Drawing for the job (mm, zero at the part's lowest x, y, z). A direction names the side the tool comes from. Round coordinates to 2 decimals unless told otherwise and drop trailing zeros. Write each loop counter-clockwise with the first axis right and the second up, starting at its lowest first coordinate (ties: lowest second). Pieces come first, ordered by that corner, then holes. Notation, with made-up numbers: (6, 33) - (30, 33) arc R27 cw to (30, 54) - close; hole circle Ø7 at (-28, -40). An arc over 180 degrees is marked (long way). Answer in a Markdown table with one row per item.
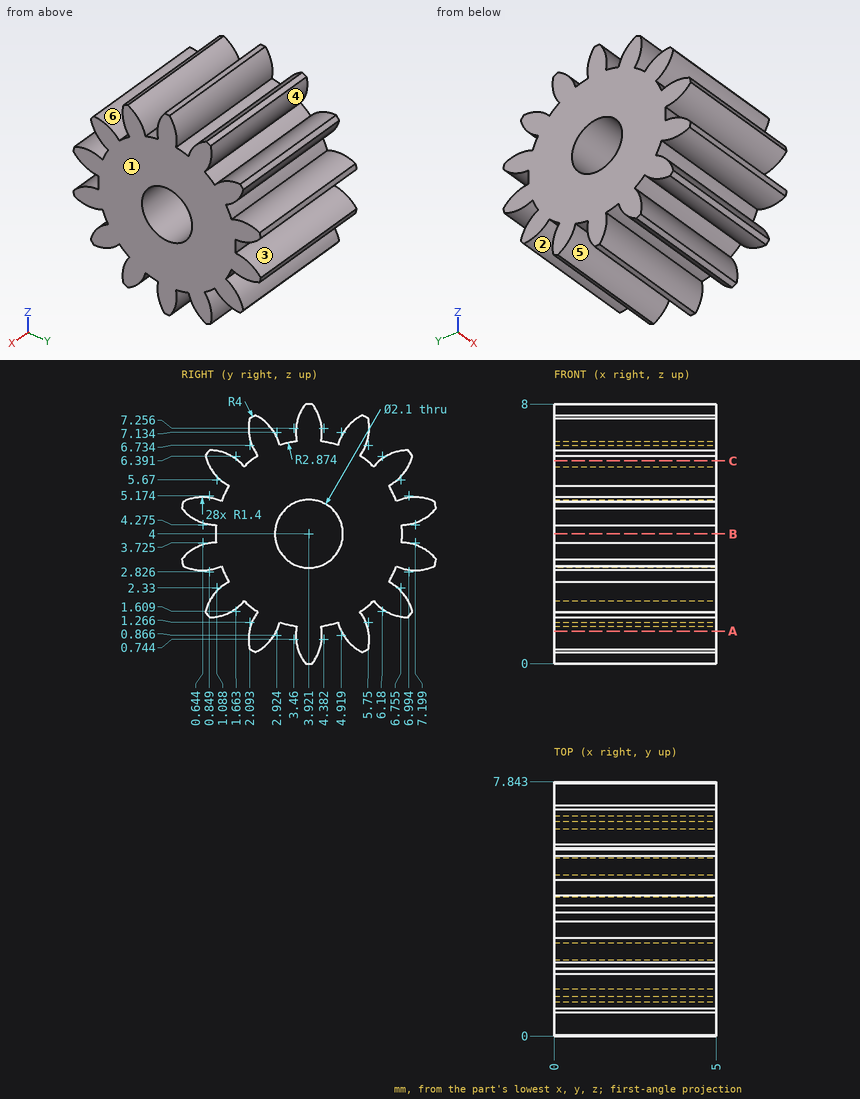
Q1. Saw through at C-C on z = 6.25. List the corners of the cut face in (x, y) (1 decimal).
Computed:
| item | result |
|---|---|
| outline | (0, 0.8) - (5, 0.8) - (5, 1.7) - (0, 1.7) - close; (0, 2.1) - (5, 2.1) - (5, 5.7) - (0, 5.7) - close; (0, 6.1) - (5, 6.1) - (5, 7.1) - (0, 7.1) - close |
Q2. Pull direction Z, two halves, no side cores. Call the marked faces 1, 2 and 3: released by +Z, released by -Z, zero draft, split by the parting line, or undercut.
Computed:
| item | result |
|---|---|
| face 1 | zero draft |
| face 2 | released by -Z |
| face 3 | undercut |
Q3. Flat gauge pin, fed straight in: pin 1 (3 mm diameter, centred on x = 2, z = 7, fed in from -Y). Where does the tip first touch, or does it go through?
Computed:
| item | result |
|---|---|
| pin 1 | stops at y = 0.73 |
Q4. Saw through at A-A on z = 1. List the corners of the cut face in (x, y) (1 decimal).
Computed:
| item | result |
|---|---|
| outline | (0, 2.1) - (5, 2.1) - (5, 2.9) - (0, 2.9) - close; (0, 3.5) - (5, 3.5) - (5, 4.3) - (0, 4.3) - close; (0, 4.9) - (5, 4.9) - (5, 5.8) - (0, 5.8) - close |
Q5. 3-axis set-ups, long thin cutter, end or side, ignore diameter. For the marked faces 4, 5 and 6: which of +Z, -Z, +X, -X, +Y, -Y reach the whole face in a straight line?
Computed:
| item | result |
|---|---|
| face 4 | +X, -X |
| face 5 | -Z, +X, -X |
| face 6 | +Z, +X, -X |
Q6. Drill centre lines: line 1 (Y direction, x = 0.95, z = 7.25) (1 decimal); line 2 (Y direction, x = 3.1, z = 4) (1 decimal); line 3 (Z direction, x = 4.75, y = 1) (1 decimal). Where is each one in solid material? Low to high.
Computed:
| item | result |
|---|---|
| line 1 | y = 2.1 to 2.8, 3.5 to 4.3, 5.1 to 5.8 |
| line 2 | y = 1 to 2.9, 5 to 6.8 |
| line 3 | z = 1.4 to 2.1, 2.9 to 3.7, 4.3 to 5.1, 5.9 to 6.6 |
Q7. Saw through at B-B on z = 4. List the corners of the cut face in (x, y) (1 decimal).
Computed:
| item | result |
|---|---|
| outline | (0, 1) - (5, 1) - (5, 2.9) - (0, 2.9) - close; (0, 5) - (5, 5) - (5, 6.8) - (0, 6.8) - close |
